The drawing under review shows one solid part. Ordinate dimensions are in mm from its lowest x, y, z. Round coordinates to 2 decimals unless told otherwise and drop trailing zeros. Order: outer loops, then holes, each group sorted by start corner. A loop starts at its lowest first (then second) coordinate and runs counter-clockwise, first axis right, second up. Notation, with made-up numbers: (3, 3.5) -> (55, 3.5) arc R19 cw to (55, 32.5) -> close; hole circle Ø10 at (69.25, 43.25). An arc over 180 degrees is marked (long way). Use a Markdown table: item, result. Add a question column.
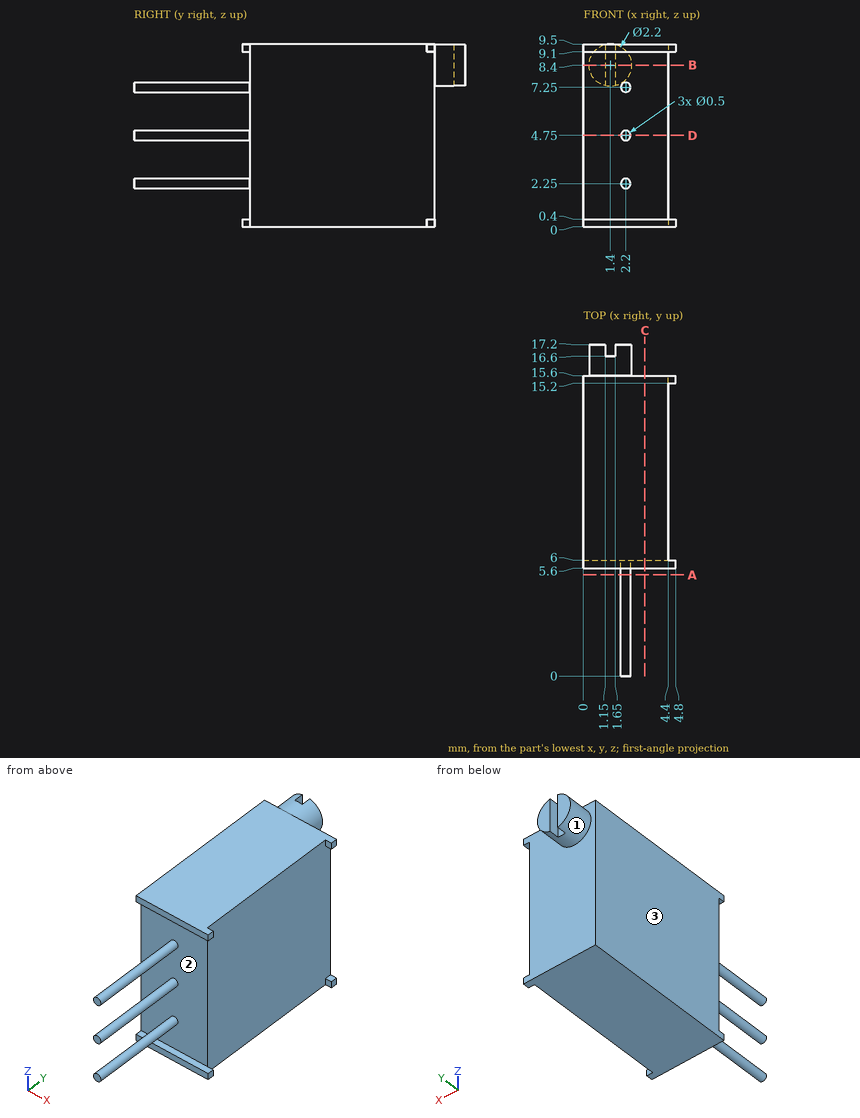
Q1. Add section D-D, the plane z = 4.75. Give the boundary of the cut face in (x, y), then the cut area to 3 significant figures.
Q2. For pin 1 (1.3 mm diameter, centred on x = 1.5, z = 5.5, fed in from -Y); pin 2 (0.7 mm diameter, centred on y = 17, z = 8.5, fed in from +X); pin 3 (0.5 mm diameter, centred on y = 17, z = 8.5, fed in from -X); pin 4 (0.6 mm diameter, centred on x = 1.5, z = 8.5, fed in from +Y), all flat-tipped, find the tip position at first contact; note any pin that passes through.
Q3. To check wall thickness, follow line 1 along X through (y, z) = (6.25, 8.5); line 2 along Y through (x, z) = (2, 1.75); line 3 along X through (y, z) = (1.25, 2.25). State the ranges of each line that lie inside material, in increasing order.
Q4. Add section C-C, the plane x = 3.2. Give the boundary of the cut face in (y, z), then the cut area to 3 significant figures.
Q5. Add section A-A, the plane y = 5.25. Give the boundary of the cut face in (x, z), then the cut area to 3 significant figures.
Q6. Add section B-B, the plane z = 8.4. Give the boundary of the cut face in (x, y).
Q7. Draft analysis for pull direction Z (two halves, no side actions). For the marked faces 1, 2 and 3, state which applies: released by +Z, released by -Z, zero draft, split by the parting line, or undercut.
Return value:
| question | item | result |
|---|---|---|
| 1 | outline | (0, 6) -> (1.95, 6) -> (1.95, 0) -> (2.45, 0) -> (2.45, 6) -> (4.4, 6) -> (4.4, 15.6) -> (0, 15.6) -> close |
| 1 | area | 45.2 mm² |
| 2 | pin 1 | y = 6 |
| 2 | pin 2 | x = 2.5 |
| 2 | pin 3 | x = 0.3 |
| 2 | pin 4 | y = 17.2 |
| 3 | line 1 | 0 to 4.4 |
| 3 | line 2 | 6 to 15.6 |
| 3 | line 3 | 1.95 to 2.45 |
| 4 | outline | (5.6, 0) -> (15.6, 0) -> (15.6, 9.5) -> (5.6, 9.5) -> (5.6, 9.1) -> (6, 9.1) -> (6, 0.4) -> (5.6, 0.4) -> close |
| 4 | area | 91.5 mm² |
| 5 | outline | circle Ø0.5 at (2.2, 2.25); circle Ø0.5 at (2.2, 4.75); circle Ø0.5 at (2.2, 7.25) |
| 5 | area | 0.589 mm² |
| 6 | outline | (0, 6) -> (4.4, 6) -> (4.4, 15.6) -> (2.5, 15.6) -> (2.5, 17.2) -> (1.65, 17.2) -> (1.65, 16.6) -> (1.15, 16.6) -> (1.15, 17.2) -> (0.3, 17.2) -> (0.3, 15.6) -> (0, 15.6) -> close |
| 7 | face 1 | split by the parting line |
| 7 | face 2 | undercut |
| 7 | face 3 | zero draft |
